CAD build for the part. Positions are in the model's coordinates, mm. Face numbers are marked on the shaded views. A direction names the side the tool comes from. Give positions to 0.01 mm unless a question says otherwise; leave off trailing zeros. Write each loop counter-clockwise with the first axis right and the second up, starting at its lowest first coordinate (ties: lowest second). Pieces come first, ordered by that corner, then holes. Notation, with made-up numbers: (55.25, 11.5) - (60.25, 11.5) arc R19 ccw to (60.25, 20.5) - close; hole circle Ø10 at (78, 88). An arc over 180 degrees is marked (long way). Answer as a JSON object with one key per item and string values.
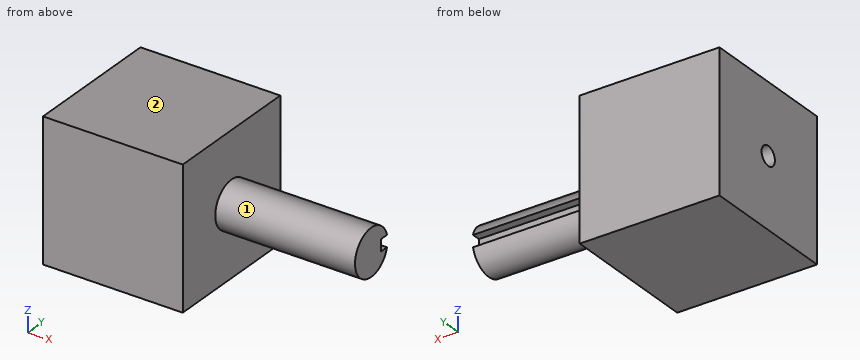
Autodesk Inventor part; units mm, degrees
ref_plane "YZ Plane" through (0, 0, 0) normal (1, 0, 0) x (0, 1, 0)
ref_plane "XZ Plane" through (0, 0, 0) normal (0, 1, 0) x (-1, 0, 0)
ref_plane "XY Plane" through (0, 0, 0) normal (0, 0, 1) x (1, 0, 0)
sketch "Sketch1" plane through (0, 0, 0) normal (0, 0, 1) x (1, 0, 0)
  line L0 (-38.1, 0) -> (0, 0)
  line L1 (0, 0) -> (0, 38.1)
  line L2 (0, 38.1) -> (-38.1, 38.1)
  line L3 (-38.1, 38.1) -> (-38.1, 0)
  dimension "d0" = 38.1
  dimension "d1" = 38.1
extrude "Extrusion1" add sketch "Sketch1" along normal blind 38.1
sketch "Sketch2" plane through (0, 0, 0) normal (1, 0, 0) x (0, 0, -1)
  line L0 (-38.1, 38.1) -> (-38.1, 0)
  line L1 (0, 0) -> (-38.1, 0)
  line L2 (0, 0) -> (0, 38.1)
  line L3 (0, 38.1) -> (-38.1, 38.1)
  line L4 (-38.1, 38.1) -> (-38.1, 0)
  line L5 (0, 0) -> (-38.1, 0)
  line L6 (0, 0) -> (0, 38.1)
  line L7 (0, 38.1) -> (-38.1, 38.1)
  circle A0 centre (-19.05, 19.05) radius 6.35
  dimension "d4" = 19.05
  dimension "d5" = 12.7
sketch "Sketch3" plane through (0, 0, 0) normal (1, 0, 0) x (0, 0, -1)
  line L0 (0, 38.1) -> (-38.1, 38.1)
  circle A0 centre (-19.05, 19.05) radius 6.35
  line L1 (-20.6502, 25.1951) -> (-20.6502, 22.86)
  line L2 (-20.6502, 22.86) -> (-17.4752, 22.86)
  line L3 (-17.4752, 22.86) -> (-17.4752, 25.2016)
  point P0 (-19.05, 25.4)
  dimension "d6" = 1.6002
  dimension "d7" = 3.175
  dimension "d8" = 1.6002
  dimension "d9" = 2.54
extrude "Extrusion2" add sketch "Sketch3" along normal blind 38.1 contours A0 L1 L2 L3 picked at (-18.8789, 19.481)
sketch "Sketch4" plane through (-38.1, 0, 0) normal (-1, 0, 0) x (0, 0, 1)
  line L0 (38.1, 0) -> (38.1, 38.1)
  line L1 (0, 0) -> (38.1, 0)
  circle A0 centre (19.05, 19.05) radius 2.6035
  dimension "d12" = 19.05
  dimension "d13" = 19.05
  dimension "d14" = 5.207
extrude "Extrusion3" cut sketch "Sketch4" against normal blind 7.747
properties part number "BaneBots P60 4 to1 gearbox"
(1) 3-axis set-ups, long thin cutter, end or side, ignore diameter. For the marked faces 1 and 2: which of +Z, -Z, +X, -X, +Y, -Y reach the whole face in a straight line?
Answer key:
{"face 1": "+X", "face 2": "+Z, +X, -X, +Y, -Y"}
(2) Saw through at C-C, the plane z = 32. Give the cut face in (x, y).
Answer key:
{"outline": "(-38.1, 0) - (0, 0) - (0, 38.1) - (-38.1, 38.1) - close"}
(3) Saw through at D-D, the plane x = 16.5. Give the cut face in (y, z), and give its area (3 significant figures).
Answer key:
{"outline": "(22.86, 17.48) - (22.86, 20.65) - (25.2, 20.65) arc R6.35 ccw (long way) to (25.2, 17.48) - close", "area": "119 mm²"}
(4) Probe L1, parallel to Y at x = -32, z = 19; L2, parallel to X at y = 7.5, z = 27.5; L3, parallel to Y at x = 31, z = 21. List the from-to ranges inside material, lowest first. Write a range as [from, to].
Answer key:
{"L1": "y = [0, 16.45], [21.65, 38.1]", "L2": "x = [-38.1, 0]", "L3": "y = [13.01, 25.09]"}
(5) Saw through at B-B, the plane y = 19.05. Give the cut face in (x, z).
Answer key:
{"outline": "(-38.1, 0) - (0, 0) - (0, 12.7) - (38.1, 12.7) - (38.1, 25.4) - (0, 25.4) - (0, 38.1) - (-38.1, 38.1) - (-38.1, 21.65) - (-30.35, 21.65) - (-30.35, 16.45) - (-38.1, 16.45) - close"}
(6) Saw through at A-A, the plane z = 19.05. Give the cut face in (x, y), and give its area (3 significant figures).
Answer key:
{"outline": "(-38.1, 0) - (0, 0) - (0, 12.7) - (38.1, 12.7) - (38.1, 22.86) - (0, 22.86) - (0, 38.1) - (-38.1, 38.1) - (-38.1, 21.65) - (-30.35, 21.65) - (-30.35, 16.45) - (-38.1, 16.45) - close", "area": "1,800 mm²"}
(7) Flat gauge pins, fed straight in: P1, Ø7, axis at y = 19.05, z = 19.05, coming from the -X side; P2, Ø1.9, axis at x = 18, y = 24.5, coming from the +Z side; P3, Ø1.6, axis at x = 16.5, z = 19, coming from the +Y side; P4, Ø2.5, axis at x = 21, y = 24, coming from the -Z side. Where does each tip first touch, or does it go through?
Answer key:
{"P1": "stops at x = -38.1", "P2": "stops at z = 23.53", "P3": "stops at y = 22.86", "P4": "stops at z = 13.89"}
